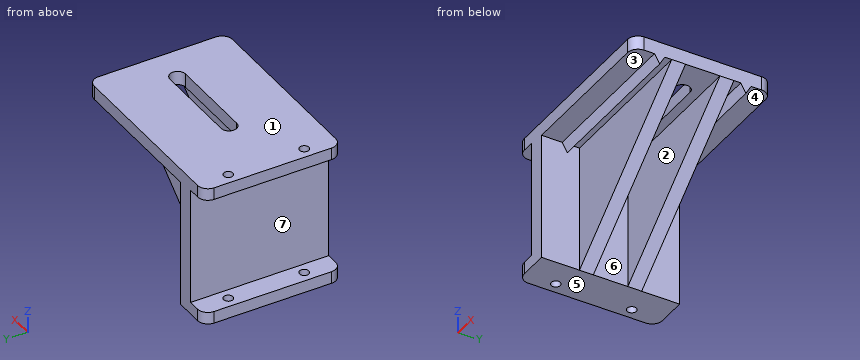
```python
from build123d import *

# Parameters (mm, degrees)
SKETCH_1_W               = 41
SKETCH_1_H               = 40
EXTRUDE_1_DEPTH          = 5
SKETCH_2_W               = 3.5
SKETCH_2_H               = 40
EXTRUDE_2_DEPTH          = 6.4
EXTRUDE_3_DEPTH          = 45
SKETCH_4_W               = 45
SKETCH_4_H               = 4
EXTRUDE_4_DEPTH          = 37
CUT_EXTRUDE_1_DEPTH      = 19
SKETCH_6_R               = 1.35
CUT_EXTRUDE_2_DEPTH      = 42
FILLET_1_R               = 3
FILLET_2_R               = 3
CUT_EXTRUDE_3_DEPTH      = 38
CUT_EXTRUDE_3_DEPTH_BACK = 5


with BuildPart() as part:
    # 스케치1 → 보스-돌출1 (new body)
    with BuildSketch(Plane(origin=(0, 0, 0), x_dir=(0, 0, -1), z_dir=(1, 0, 0))):
        with Locations((20.5, 20)):
            Rectangle(SKETCH_1_W, SKETCH_1_H)
    extrude(amount=EXTRUDE_1_DEPTH)

    # 스케치2 → 보스-돌출2 (add)
    with BuildSketch(Plane.ZY):
        with Locations((-1.75, 20)):
            Rectangle(SKETCH_2_W, SKETCH_2_H)
        with Locations((-39.25, 20)):
            Rectangle(SKETCH_2_W, SKETCH_2_H)
    extrude(amount=EXTRUDE_2_DEPTH)

    # 스케치3 → 보스-돌출3 (add)
    with BuildSketch(Plane(origin=(5, 0, 0), x_dir=(0, 0, -1), z_dir=(1, 0, 0))):
        Polygon((0, 40), (4, 40), (4, 34), (6.598076211, 32.5), (4, 31), (4, 14), (4, 12), (4, 9), (6.598076211, 7.5), (4, 6), (4, 0), (0, 0), align=None)
    extrude(amount=EXTRUDE_3_DEPTH)

    # 스케치4 → 보스-돌출4 (add)
    with BuildSketch(Plane(origin=(0, 0, -4), x_dir=(-1, 0, 0), z_dir=(0, 0, -1))):
        with Locations((-27.5, 27)):
            Rectangle(SKETCH_4_W, SKETCH_4_H)
        with Locations((-27.5, 13)):
            Rectangle(SKETCH_4_W, SKETCH_4_H)
    extrude(amount=EXTRUDE_4_DEPTH)

    # 스케치5 → 컷-돌출1 (cut)
    with BuildSketch(Plane(origin=(0, 29, 0), x_dir=(1, 0, 0), z_dir=(0, 1, 0))):
        Polygon((50, 4), (5, 41), (50, 41), align=None)
    extrude(amount=-CUT_EXTRUDE_1_DEPTH, mode=Mode.SUBTRACT)

    # 스케치6 → 컷-돌출2 (cut, through all)
    with BuildSketch(Plane(origin=(0, 0, -41), x_dir=(-1, 0, 0), z_dir=(0, 0, -1))):
        with Locations((3.2, 9)):
            Circle(SKETCH_6_R)
        with Locations((3.2, 31)):
            Circle(SKETCH_6_R)
    extrude(amount=-CUT_EXTRUDE_2_DEPTH, mode=Mode.SUBTRACT)

    # 필렛1
    fillet_1_edges = [part.edges().sort_by_distance(p)[0] for p in [
        (50, 0, -2),
        (50, 40, -2),
    ]]
    fillet(fillet_1_edges, radius=FILLET_1_R)

    # 필렛2
    fillet_2_edges = [part.edges().sort_by_distance(p)[0] for p in [
        (-6.4, 0, -1.75),
        (-6.4, 40, -1.75),
        (-6.4, 40, -39.25),
        (-6.4, 0, -39.25),
    ]]
    fillet(fillet_2_edges, radius=FILLET_2_R)

    # 스케치7 → 컷-돌출3 (cut, two sides)
    with BuildSketch(Plane(origin=(0, 0, -4), x_dir=(-1, 0, 0), z_dir=(0, 0, -1))) as cut_extrude_3_sk:
        with BuildLine():
            Line((-40, 22.25), (-15, 22.25))
            ThreePointArc((-15, 22.25), (-12.75, 20), (-15, 17.75))
            Line((-15, 17.75), (-40, 17.75))
            ThreePointArc((-40, 17.75), (-42.25, 20), (-40, 22.25))
        make_face()
    extrude(amount=CUT_EXTRUDE_3_DEPTH, mode=Mode.SUBTRACT)
    extrude(cut_extrude_3_sk.sketch, amount=-CUT_EXTRUDE_3_DEPTH_BACK, mode=Mode.SUBTRACT)


solid = part.part
```
The model under review builds one solid part; all positions refer to its coordinate system, in mm. Face numbers are marked on the shaded views. A direction names the side the tool comes from. Round coordinates to 2 decimals unless told otherwise and drop trailing zeros. Write each loop counter-clockwise with the first axis right and the second up, starting at its lowest first coordinate (ties: lowest second). Pieces come first, ordered by that corner, then holes.
(1) We need section C-C on z = -8. Give the boundary of the cut face in (x, y), and give its area (3 significant figures).
(2) Machinability: for the marked faces 1, 2, 3 and 4, which of the approach directions +Z, -Z, +X, -X, +Y, -Y give a long, thin tool a straight path to every point of the face, cutting with its end or side? Answer none if there is none.
(3) Insertion check: pin 1 (5 mm diameter, centred on x = 22, y = 20.5, fed in from -Z); pin 2 (3.5 mm diameter, centred on y = 3, z = -25.5, fed in from +X); pin 3 (10 mm diameter, centred on x = 36.5, y = 35.5, fed in from -Z). Each pin has a flat end and moves straight along its axis. Give the tip position at first contact, or say it passes through.
(4) Mouldability with a two-part tool opening along Z and no side actions: class the marked faces 5, 6 and 7 as +Z half, -Z half, draft (parallel to the pull), parting line (faces both ways), or undercut.
(5) Wall thickness on L1, parallel to Y at x = -3.2, z = -38.75; L2, parallel to Y at x = 10.5, z = -17; L3, parallel to Y at x = 37.5, z = -3.5: over which ranges is each line inside the solid? List them lowest first.
(6) We need section B-B on y = 20. Give the boundary of the cut face in (x, z).
(7) We need section A-A on x = 24. Give the boundary of the cut face in (y, z).
(8) We need section D-D on z = -21.5. Give the boundary of the cut face in (x, y), and give its area (3 significant figures).
Findings below:
1. outline: (0, 0) - (5, 0) - (5, 11) - (45.14, 11) - (45.14, 15) - (5, 15) - (5, 25) - (45.14, 25) - (45.14, 29) - (5, 29) - (5, 40) - (0, 40) - close
1. area: 521 mm2
2. face 1: +Z, +X, -X, +Y, -Y
2. face 2: -Z, +X
2. face 3: -Z, +X, -Y
2. face 4: -Z, +X, +Y
3. pin 1: stops at z = -4
3. pin 2: stops at x = 5
3. pin 3: stops at z = -6.6
4. face 5: -Z half
4. face 6: draft
4. face 7: undercut
5. L1: y = 0 to 7.65, 10.35 to 29.65, 32.35 to 40
5. L2: y = 11 to 15, 25 to 29
5. L3: y = 0 to 17.75, 22.25 to 40
6. outline: (-6.4, -41) - (5, -41) - (5, -4) - (12.75, -4) - (12.75, 0) - (-6.4, 0) - (-6.4, -3.5) - (0, -3.5) - (0, -37.5) - (-6.4, -37.5) - close; (42.25, -4) - (50, -4) - (50, 0) - (42.25, 0) - close
7. outline: (0, -4) - (6, -4) - (7.5, -6.6) - (9, -4) - (11, -4) - (11, -25.38) - (15, -25.38) - (15, -4) - (17.75, -4) - (17.75, 0) - (0, 0) - close; (22.25, -4) - (25, -4) - (25, -25.38) - (29, -25.38) - (29, -4) - (31, -4) - (32.5, -6.6) - (34, -4) - (40, -4) - (40, 0) - (22.25, 0) - close
8. outline: (0, 0) - (5, 0) - (5, 11) - (28.72, 11) - (28.72, 15) - (5, 15) - (5, 25) - (28.72, 25) - (28.72, 29) - (5, 29) - (5, 40) - (0, 40) - close
8. area: 390 mm2
